Geometry: final body of the model. Coordinates: model frame, mm. Face numbers are marked on the shaded views. A direction names the side the tool comes from. Give positions to 0.01 mm unless a question says otherwise; leave off trailing zeros. Loops run counter-clockwise (first coordinate to the right, second up) from the corner with the lowest first, then second, coordinate; pieces in that order, holes last. Notation, with made-up numbers: (31, -37.5) -> (52, -37.5) arc R32 cw to (52, -7.5) -> close; hole circle Ø5 at (-10.5, 73.5). An arc over 180 degrees is marked (long way). Answer in a Markdown table with one row per item. Add a question column.
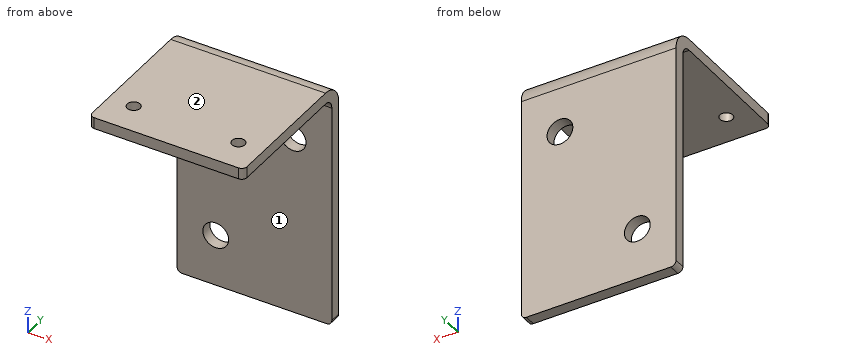
from build123d import *

# Parameters (mm, degrees)
F1_DEPTH = 38.1
F2_R     = 1.27
F3_R     = 1.5875
F4_DEPTH = 2.794
F5_R     = 3.175
F6_DEPTH = 2.794


with BuildPart() as f1:
    # F0 (on Right) → F1 (new body)
    with BuildSketch(Plane.YZ):
        with BuildLine():
            Line((-2.794, 0), (0, 0))
            Line((0, 0), (0, 55.626))
            ThreePointArc((0, 55.626), (-1.562292, 59.397708), (-5.334, 60.96))
            Line((-5.334, 60.96), (-38.354, 60.96))
            Line((-38.354, 60.96), (-38.354, 58.166))
            Line((-38.354, 58.166), (-5.334, 58.166))
            ThreePointArc((-5.334, 58.166), (-3.537949, 57.422051), (-2.794, 55.626))
            Line((-2.794, 55.626), (-2.794, 0))
        make_face()
    extrude(amount=F1_DEPTH)

    # F2
    f2_edges = [f1.edges().sort_by_distance(p)[0] for p in [
        (0, -38.354, 59.563),
        (38.1, -38.354, 59.563),
        (38.1, -1.397, 0),
        (0, -1.397, 0),
    ]]
    fillet(f2_edges, radius=F2_R)

    # F3 (on face) → F4 (cut, through all)
    with BuildSketch(Plane.XY.offset(60.96)):
        with Locations((31.9405, -30.4038)):
            Circle(F3_R)
        with Locations((6.1595, -30.4038)):
            Circle(F3_R)
    extrude(amount=-F4_DEPTH, mode=Mode.SUBTRACT)

    # F5 (on face) → F6 (cut, through all)
    with BuildSketch(Plane.XZ.offset(2.794)):
        with Locations((28.575, 44.5008)):
            Circle(F5_R)
        with Locations((9.525, 12.7508)):
            Circle(F5_R)
    extrude(amount=-F6_DEPTH, mode=Mode.SUBTRACT)


solid = f1.part
(1) Pin query (flat end, axial travel): pin 1 Ø4 at (x, y) = (17, -24.5) entering from -Z; pin 2 Ø1.5 at (x, z) = (12, 52.5) entering from -Y; pin 3 Ø12 at (x, z) = (18, 50.5) entering from -Y. Return the tip coordinate at first contact, or that it passes through.
(2) Cut plane A-A on x = 35.5. Return the cut outline in (y, z), then the cut area to 3 significant figures.
(3) Reachability of the marked faces 1 and 2 from +Z, -Z, +X, -X, +Y, -Y: full face, straight path, thin tool, end or side. Return the list, or none.
(4) Cut plane C-C on x = 29. Return the cut outline in (y, z), then the cut area to 3 significant figures.
(5) Cut plane B-B on z = 15. Return the cut outline in (x, y).
(6) Material intervals for line 1 along Z through (x, y) = (32, -9); line 2 along Y through (x, z) = (27.5, 24); line 3 along Z through (x, y) = (5, -4), sorted ascending. Write a range as from..to.
(7) Cut plane D-D on y = -17.5. Return the cut outline in (x, z).
Answer list:
| question | item | result |
|---|---|---|
| 1 | pin 1 | stops at z = 58.17 |
| 1 | pin 2 | stops at y = -2.79 |
| 1 | pin 3 | stops at y = -2.95 |
| 2 | outline | (-38.35, 58.17) -> (-5.33, 58.17) arc R2.54 cw to (-2.79, 55.63) -> (-2.79, 0) -> (0, 0) -> (0, 55.63) arc R5.33 ccw to (-5.33, 60.96) -> (-38.35, 60.96) -> close |
| 2 | area | 265 mm² |
| 3 | face 1 | -Z, +X, -X, -Y |
| 3 | face 2 | +Z, +X, -X, +Y, -Y |
| 4 | outline | (-38.35, 58.17) -> (-5.33, 58.17) arc R2.54 cw to (-2.79, 55.63) -> (-2.79, 47.65) -> (0, 47.65) -> (0, 55.63) arc R5.33 ccw to (-5.33, 60.96) -> (-38.35, 60.96) -> close; (-2.79, 0) -> (0, 0) -> (0, 41.35) -> (-2.79, 41.35) -> close |
| 4 | area | 247 mm² |
| 5 | outline | (0, -2.79) -> (7.28, -2.79) -> (7.28, 0) -> (0, 0) -> close; (11.77, -2.79) -> (38.1, -2.79) -> (38.1, 0) -> (11.77, 0) -> close |
| 6 | line 1 | z = 58.17..60.96 |
| 6 | line 2 | y = -2.79..0 |
| 6 | line 3 | z = 57.79..60.79 |
| 7 | outline | (0, 58.17) -> (38.1, 58.17) -> (38.1, 60.96) -> (0, 60.96) -> close |
